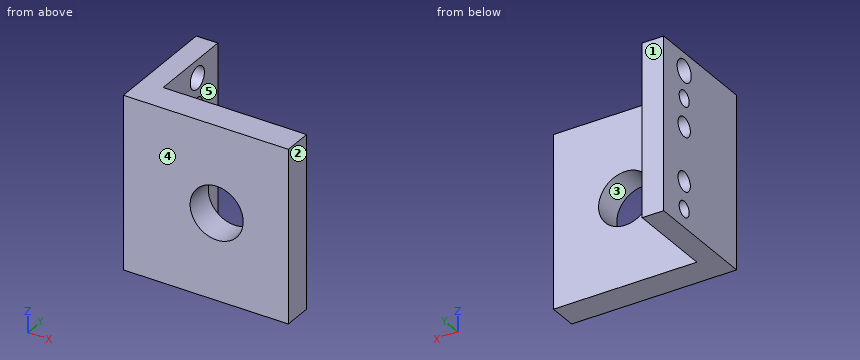
```python
from build123d import *

# Parameters (mm, degrees)
SKETCH_1_W      = 20
SKETCH_1_H      = 24
SKETCH_1_R      = 3.7
EXTRUDE_1_DEPTH = 4
SKETCH_2_W      = 24
SKETCH_2_H      = 16
SKETCH_2_R      = 1.1
SKETCH_2_R_2    = 1.35
SKETCH_2_R_3    = 1.55
EXTRUDE_2_DEPTH = 3


with BuildPart() as part:
    # 草图1 → 凸台-拉伸1 (new body)
    with BuildSketch(Plane(origin=(0, 0, 0), x_dir=(1, 0, 0), z_dir=(0, 1, 0))):
        with Locations((10, 12)):
            Rectangle(SKETCH_1_W, SKETCH_1_H)
        with Locations(Location((10, 12, 0), (0, 0, 270))):
            Circle(SKETCH_1_R, mode=Mode.SUBTRACT)
    extrude(amount=EXTRUDE_1_DEPTH)

    # 草图2 → 凸台-拉伸2 (add)
    with BuildSketch(Plane.ZY):
        with Locations((-12, 8)):
            Rectangle(SKETCH_2_W, SKETCH_2_H)
        with Locations((-21.5, 11.5)):
            Circle(SKETCH_2_R, mode=Mode.SUBTRACT)
        with Locations((-17.7, 11.5)):
            Circle(SKETCH_2_R_2, mode=Mode.SUBTRACT)
        with Locations((-6.3, 11.5)):
            Circle(SKETCH_2_R, mode=Mode.SUBTRACT)
        with Locations((-2.5, 11.5)):
            Circle(SKETCH_2_R_3, mode=Mode.SUBTRACT)
        with Locations((-10.2, 11.5)):
            Circle(SKETCH_2_R_2, mode=Mode.SUBTRACT)
    extrude(amount=EXTRUDE_2_DEPTH)


solid = part.part
```
The model under review builds one solid part; all positions refer to its coordinate system, in mm. Face numbers are marked on the shaded views. A direction names the side the tool comes from. Coordinates: 2 decimals unless noted, no trailing zeros. Write each loop counter-clockwise with the first axis right and the second up, starting at its lowest first coordinate (ties: lowest second). Pieces come first, ordered by that corner, then holes. Notation, with made-up numbers: (55, -2) -> (70, -2) arc R35 cw to (70, 31) -> close; hole circle Ø1 at (-9.75, 44). An arc over 180 degrees is marked (long way). One line per item, written item: value. Start each with the question number.
Q1. Clearance check with flat-ended pins moving along their axes: P1, Ø3.5, axis at y = 11.5, z = -6.3, coming from the -X side; P2, Ø5, axis at y = 12, z = -12, coming from the +X side; P3, Ø9.5, axis at x = 10, z = -12, coming from the +Y side; P4, Ø2, axis at y = 11.5, z = -10.2, coming from the -X side. State where each tip first meets the part, or that it passes through.
Q2. To check wall thickness, follow probe 1 along Y at (x, z) = (-1.45, -21.5); probe 2 along Y at (x, z) = (-2.05, -2.5); probe 3 along Y at (x, z) = (14, -12). State the ranges of each line that lie inside material, in increasing order.
Q3. Add section D-D, the plane z = -9.75. Give the boundary of the cut face in (x, y).
Q4. Add section A-A, the plane z = -2.5. Give the boundary of the cut face in (x, y).
Q5. Add section B-B, the plane y = 11.5. Give the boundary of the cut face in (x, z), then the cut area to 3 significant figures.
Q6. For the marked faces 4 and 5, list the 3-axis set-ups (+Z, -Z, +X, -X, +Y, -Y) from which the entire face can be reached by the end or side of a thin tool; tool diameter is ignored.
Q7. Add section C-C, the plane x = 10. Give the boundary of the cut face in (y, z), then the cut area to 3 significant figures.
Q8. The part is to be moulded in two halves that separate along X. For the marked faces 1, 2 and 3, say which applies: +X half, -X half, draft (parallel to the pull), parting line (faces both ways), or undercut.
Response:
1. P1: x = -3
1. P2: x = 0
1. P3: y = 4
1. P4: through
2. probe 1: 0 to 10.4, 12.6 to 16
2. probe 2: 0 to 9.95, 13.05 to 16
2. probe 3: 0 to 4
3. outline: (-3, 0) -> (7.06, 0) -> (7.06, 4) -> (0, 4) -> (0, 10.23) -> (-3, 10.23) -> close; (-3, 12.77) -> (0, 12.77) -> (0, 16) -> (-3, 16) -> close; (12.94, 0) -> (20, 0) -> (20, 4) -> (12.94, 4) -> close
4. outline: (-3, 0) -> (20, 0) -> (20, 4) -> (0, 4) -> (0, 9.95) -> (-3, 9.95) -> close; (-3, 13.05) -> (0, 13.05) -> (0, 16) -> (-3, 16) -> close
5. outline: (-3, -24) -> (0, -24) -> (0, -22.6) -> (-3, -22.6) -> close; (-3, -20.4) -> (0, -20.4) -> (0, -19.05) -> (-3, -19.05) -> close; (-3, -16.35) -> (0, -16.35) -> (0, -11.55) -> (-3, -11.55) -> close; (-3, -8.85) -> (0, -8.85) -> (0, -7.4) -> (-3, -7.4) -> close; (-3, -5.2) -> (0, -5.2) -> (0, -4.05) -> (-3, -4.05) -> close; (-3, -0.95) -> (0, -0.95) -> (0, 0) -> (-3, 0) -> close
5. area: 33.3 mm²
6. face 4: +Z, -Z, +X, -X, -Y
6. face 5: +Z, -Z, +X, +Y
7. outline: (0, -24) -> (4, -24) -> (4, -15.7) -> (0, -15.7) -> close; (0, -8.3) -> (4, -8.3) -> (4, 0) -> (0, 0) -> close
7. area: 66.4 mm²
8. face 1: draft
8. face 2: +X half
8. face 3: undercut
